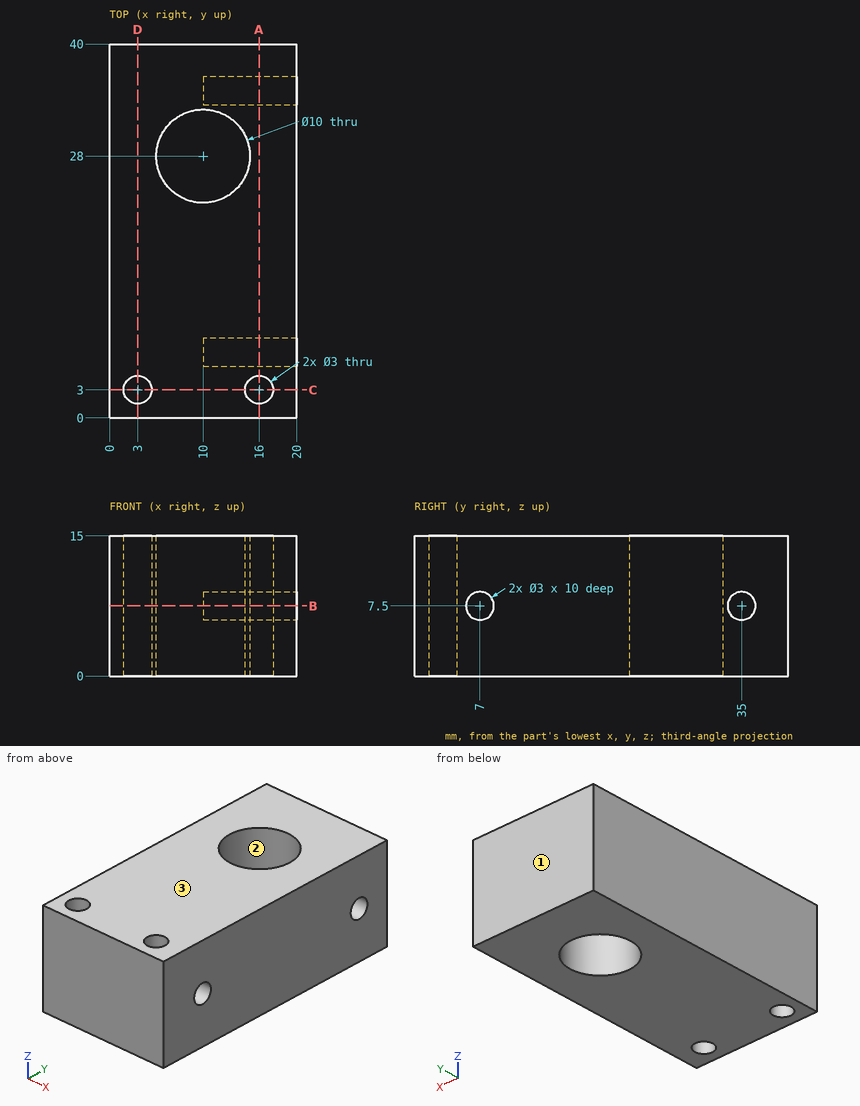
The figure shows three views and two pictorial views of one solid part (mm, origin at its lowest corner). Answer the questions. Give positions to 0.01 mm unless a question says otherwise; leave off trailing zeros. Write each loop counter-clockwise with the first axis right and the second up, starting at its lowest first coordinate (ties: lowest second). Pieces come first, ordered by that corner, then holes. Notation, with made-up numbers: (62, -30) - (81, -30) arc R30 ccw to (81, -2) - close; hole circle Ø5 at (54.25, 3). An arc over 180 degrees is marked (long way). Return JSON: item names as keys, results as strings.
Q1. Consider line 1 along Z through (x, y) = (14, 35); line 2 along Y through (x, z) = (10.25, 14); line 3 along X through (y, z) = (31.5, 11.5). Determine where each line is inside the solid, lowest interval first. Write a range as [from, to].
Reply:
{"line 1": "[0, 6], [9, 15]", "line 2": "[0, 23.01], [32.99, 40]", "line 3": "[0, 6.43], [13.57, 20]"}
Q2. A cutting plane is placed at C-C, the plane y = 3. Determine the outline of the cut face in (x, z), and give its area (3 significant figures).
Reply:
{"outline": "(0, 0) - (1.5, 0) - (1.5, 15) - (0, 15) - close; (4.5, 0) - (14.5, 0) - (14.5, 15) - (4.5, 15) - close; (17.5, 0) - (20, 0) - (20, 15) - (17.5, 15) - close", "area": "210 mm²"}
Q3. Given P1, Ø6, axis at x = 10, y = 28, coming from the +Z side; P2, Ø3.5, axis at y = 35, z = 7, coming from the +X side; P3, Ø1.8, axis at y = 35, z = 7.5, coming from the +X side, each flat-ended and moving along its own axis, determine where each tip first touches the part or whether it passes through.
Reply:
{"P1": "through", "P2": "x = 20", "P3": "x = 10"}
Q4. A cutting plane is placed at B-B, the plane z = 7.5. Determine the outline of the cut face in (x, y).
Reply:
{"outline": "(0, 0) - (20, 0) - (20, 5.5) - (10, 5.5) - (10, 8.5) - (20, 8.5) - (20, 33.5) - (10, 33.5) - (10, 36.5) - (20, 36.5) - (20, 40) - (0, 40) - close; hole circle Ø3 at (3, 3); hole circle Ø10 at (10, 28); hole circle Ø3 at (16, 3)"}
Q5. For a pull along Y with two mould halves and no side action, classify the marked faces 1, 2 and 3 as released by +Y, released by -Y, zero draft, split by the parting line, or undercut.
Reply:
{"face 1": "released by +Y", "face 2": "undercut", "face 3": "zero draft"}
Q6. A cutting plane is placed at D-D, the plane x = 3. Determine the outline of the cut face in (y, z), and give its area (3 significant figures).
Reply:
{"outline": "(0, 0) - (1.5, 0) - (1.5, 15) - (0, 15) - close; (4.5, 0) - (40, 0) - (40, 15) - (4.5, 15) - close", "area": "555 mm²"}
Q7. A cutting plane is placed at A-A, the plane x = 16. Determine the outline of the cut face in (y, z).
Reply:
{"outline": "(0, 0) - (1.5, 0) - (1.5, 15) - (0, 15) - close; (4.5, 0) - (40, 0) - (40, 15) - (4.5, 15) - close; hole circle Ø3 at (7, 7.5); hole circle Ø3 at (35, 7.5)"}
